Here's how the part is built. I have some questions about the finished solid (model axes, mm). Face numbers are marked on the shaded views. A direction names the side the tool comes from. Coordinates: 2 decimals unless noted, no trailing zeros. Order: outer loops, then holes, each group sorted by start corner. A loop starts at its lowest first (then second) coordinate and runs counter-clockwise, first axis right, second up. Notation, with made-up numbers: (73.5, 52.5) - (85.5, 52.5) arc R33 ccw to (85.5, 89.5) - close; hole circle Ø6 at (-40, 8.25). An arc over 180 degrees is marked (long way). Answer as CSV lines item,"result". Start each with the question number.
Q1. For pin 1 Ø3 at (y, z) = (2, 17.5) entering from +X; pin 2 Ø3 at (x, y) = (-27.5, -1.5) entering from +Z, each with a flat end and sliding along its axis, tell me the tip position at first contact or that it passes through.
Q2. Suppose I cut it at D-D (y = 6.75). Please give me the cut outline in (x, z).
Q3. For the marked faces 1 and 2, which set-ups out of +Z, -Z, +X, -X, +Y, -Y let a thin tool reach every point of the face, with its end or its side?
Q4. Suppose I cut it at A-A (x = 39.5). Please give me the cut outline in (y, z).
Q5. I need wall thicknesses on line 1 (Y direction, x = -41.9, z = 15); line 2 (X direction, y = 3.25, z = 14); line 3 (Z direction, x = -23.5, y = -8.25). Which ranges of each line are inside material? Lowest first, please.
Q6. Suppose I cut it at B-B (y = 0). Please give me the cut outline in (x, z).
Q7. Suppose I cut it at C-C (z = 15). Please give me the cut outline in (x, y).
from build123d import *

# Parameters (mm, degrees)
SKETCH1_W           = 89
SKETCH1_H           = 20
BOSS_EXTRUDE1_DEPTH = 5
SKETCH2_W           = 5
SKETCH2_H           = 20
BOSS_EXTRUDE2_DEPTH = 20
SKETCH3_R           = 2
CUT_EXTRUDE1_DEPTH  = 89.20997676
SKETCH4_R           = 2
CUT_EXTRUDE2_DEPTH  = 20
SKETCH5_W           = 5
SKETCH5_H           = 5
BOSS_EXTRUDE3_DEPTH = 5
CUT_EXTRUDE3_DEPTH  = 55.820160525


with BuildPart() as part:
    # Sketch1 → Boss-Extrude1 (new body)
    with BuildSketch(Plane.XY):
        Rectangle(SKETCH1_W, SKETCH1_H)
    extrude(amount=BOSS_EXTRUDE1_DEPTH)

    # Sketch2 → Boss-Extrude2 (add)
    with BuildSketch(Plane.XY.offset(5)):
        with Locations((-42, 0)):
            Rectangle(SKETCH2_W, SKETCH2_H)
    extrude(amount=BOSS_EXTRUDE2_DEPTH)

    # Sketch3 → Cut-Extrude1 (cut, through all)
    with BuildSketch(Plane(origin=(-39.5, 0, 0), x_dir=(0, 0, -1), z_dir=(1, 0, 0))):
        with Locations((-15, 0)):
            Circle(SKETCH3_R)
    extrude(amount=-CUT_EXTRUDE1_DEPTH, mode=Mode.SUBTRACT)

    # Sketch4 → Cut-Extrude2 (cut)
    with BuildSketch(Plane(origin=(0, 0, 0), x_dir=(-1, 0, 0), z_dir=(0, 0, -1))):
        with Locations((-39.5, 0)):
            Circle(SKETCH4_R)
    extrude(amount=-CUT_EXTRUDE2_DEPTH, mode=Mode.SUBTRACT)

    # Sketch5 → Boss-Extrude3 (add)
    with BuildSketch(Plane(origin=(-39.5, 0, 0), x_dir=(0, 0, -1), z_dir=(1, 0, 0))):
        with Locations((-7.5, -7.5)):
            Rectangle(SKETCH5_W, SKETCH5_H)
        with Locations((-7.5, 7.5)):
            Rectangle(SKETCH5_W, SKETCH5_H)
    extrude(amount=BOSS_EXTRUDE3_DEPTH)

    # Sketch6 → Cut-Extrude3 (cut, through all)
    with BuildSketch(Plane(origin=(0, 10, 0), x_dir=(1, 0, 0), z_dir=(0, 1, 0))):
        Polygon((-34.5, -5), (-39.5, -10), (-34.5, -10), align=None)
    extrude(amount=-CUT_EXTRUDE3_DEPTH, mode=Mode.SUBTRACT)


solid = part.part
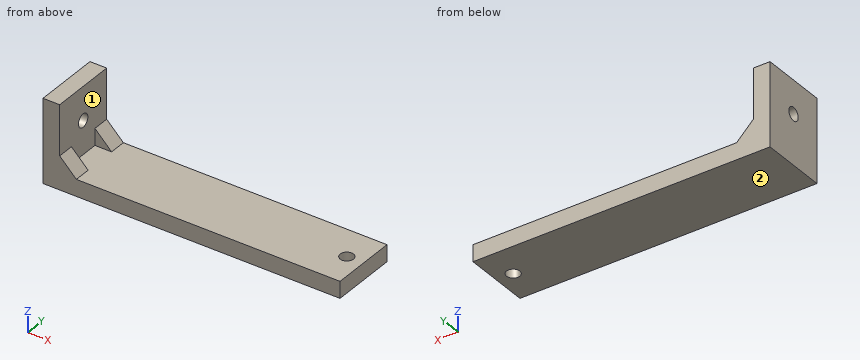
Here are the results:
1,pin 1,"stops at x = -39.5"
1,pin 2,"stops at z = 5"
2,outline,"(-44.5, 0) - (44.5, 0) - (44.5, 5) - (-34.5, 5) - (-39.5, 10) - (-39.5, 25) - (-44.5, 25) - close"
3,face 1,"+Z, +X"
3,face 2,"-Z, +X, -X, +Y, -Y"
4,outline,"(-10, 0) - (-2, 0) - (-2, 5) - (-10, 5) - close; (2, 0) - (10, 0) - (10, 5) - (2, 5) - close"
5,line 1,"y = -10 to -2, 2 to 10"
5,line 2,"x = -44.5 to -39.5"
5,line 3,"z = 0 to 5"
6,outline,"(-44.5, 0) - (37.5, 0) - (37.5, 5) - (-39.5, 5) - (-39.5, 13) - (-44.5, 13) - close; (-44.5, 17) - (-39.5, 17) - (-39.5, 25) - (-44.5, 25) - close; (41.5, 0) - (44.5, 0) - (44.5, 5) - (41.5, 5) - close"
7,outline,"(-44.5, -10) - (-39.5, -10) - (-39.5, -2) - (-44.5, -2) - close; (-44.5, 2) - (-39.5, 2) - (-39.5, 10) - (-44.5, 10) - close"
